The listing builds one solid part. Answer for the finished solid, in the listing's coordinates (mm). Face numbers are marked on the shaded views. A direction names the side the tool comes from. Round coordinates to 2 decimals unless told otherwise and drop trailing zeros. Write each loop counter-clockwise with the first axis right and the second up, starting at its lowest first coordinate (ties: lowest second). Pieces come first, ordered by that corner, then holes. Notation, with made-up numbers: (73.5, 74) - (113.5, 74) arc R19 ccw to (113.5, 80) - close; hole circle Ø10 at (36.5, 35). An arc over 180 degrees is marked (long way). Return JSON: item names as keys, results as strings. Group by question number.
(1) Which of the six approach directions +Z, -Z, +X, -X, +Y, -Y give full straight-line access (tool end or side, diameter ignored) to the marked faces 1, 2, 3, 4 and 5?
(2) Section C-C, the plane x = -25 is taken. Write down the section's boundary in (y, z), then the cut area to 3 significant figures.
(3) Section A-A, the plane z = 12.5 is taken. Write down the section's boundary in (x, y), then the cut area to 3 significant figures.
(4) Find the intervals of material crossed by line 1 along X through (y, z) = (3, 4.75); line 2 along Z through (x, y) = (-23, 33.5); line 3 along Y through (x, z) = (-60, 23.5), in increasing order. Write a range as [from, to].
(5) Section B-B, the plane y = -17 is taken. Write down the section's boundary in (x, z).
(6) Each of these flat-tipped pins is pushed along its axis until it touches: pin 1 (12.5 mm diameter, centred on y = 0.5, z = 10, fed in from -X); pin 2 (6 mm diameter, centred on x = -56.5, y = 4.5, fed in from +Z); pin 3 (6 mm diameter, centred on y = -5, z = 11, fed in from +X). Where does it stop, or does it pass through?
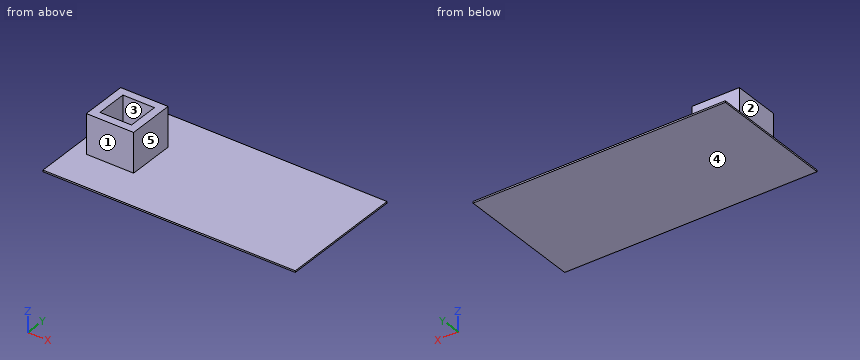
```python
from build123d import *

# Parameters (mm, degrees)
F0_W     = 160
F0_H     = 80
F1_DEPTH = 1
F2_W     = 30
F2_H     = 30
F3_DEPTH = 25
F4_W     = 20
F4_H     = 20
F5_DEPTH = 25


with BuildPart() as f1:
    # F0 (on Top) → F1 (new body)
    with BuildSketch(Plane.XY):
        Rectangle(F0_W, F0_H)
    extrude(amount=F1_DEPTH)

    # F2 (on face) → F3 (join)
    with BuildSketch(Plane.XY.offset(1)):
        with Locations((-55.679019, 0)):
            Rectangle(F2_W, F2_H)
    extrude(amount=F3_DEPTH)

    # F4 (on face) → F5 (cut)
    with BuildSketch(Plane.XY.offset(26)):
        with Locations((-55.679019, 0)):
            Rectangle(F4_W, F4_H)
    extrude(amount=-F5_DEPTH, mode=Mode.SUBTRACT)


solid = f1.part
```
Working result:
{
 "1": {"face 1": "+Z, +X, -X, -Y", "face 2": "+Z, -X, +Y, -Y", "face 3": "+Z", "face 4": "-Z, +X, -X, +Y, -Y", "face 5": "+Z, +X, +Y, -Y"},
 "2": {"outline": "(-40, 0) - (40, 0) - (40, 1) - (-40, 1) - close", "area": "80.0 mm^2"},
 "3": {"outline": "(-70.68, -15) - (-40.68, -15) - (-40.68, 15) - (-70.68, 15) - close; hole (-65.68, -10) - (-45.68, -10) - (-45.68, 10) - (-65.68, 10) - close", "area": "500 mm^2"},
 "4": {"line 1": "x = [-70.68, -65.68], [-45.68, -40.68]", "line 2": "z = [0, 1]", "line 3": "y = [-15, -10], [10, 15]"},
 "5": {"outline": "(-80, 0) - (80, 0) - (80, 1) - (-80, 1) - close"},
 "6": {"pin 1": "stops at x = -70.68", "pin 2": "stops at z = 1", "pin 3": "stops at x = -40.68"}
}
